Read the model definition and answer for the solid it produces. Units are mm, in the model's axes. A direction names the side the tool comes from. Coordinates: 2 decimals unless noted, no trailing zeros. Loops run counter-clockwise (first coordinate to the right, second up) from the corner with the lowest first, then second, coordinate; pieces in that order, holes last.
from build123d import *

# Parameters (mm, degrees)
SKETCH1_R           = 2.1209
SKETCH1_R_2         = 1.6002
BOSS_EXTRUDE1_DEPTH = 4.7625
CUT_EXTRUDE1_DEPTH  = 37.357096109
FILLET1_R           = 0.79375


with BuildPart() as part:
    # Sketch1 → Boss-Extrude1 (new body)
    with BuildSketch(Plane(origin=(0, 0, 0), x_dir=(0, 0, -1), z_dir=(1, 0, 0))):
        with BuildLine():
            ThreePointArc((-3.890248837, 27.252752244), (0, 34.7625), (3.890248837, 27.252752244))
            ThreePointArc((3.890248837, 27.252752244), (2.38125, 22.5), (3.890248837, 17.747247756))
            ThreePointArc((3.890248837, 17.747247756), (4.735348571, 15.507819022), (4.384317755, 13.140117187))
            ThreePointArc((4.384317755, 13.140117187), (4.159430641, 10.081636558), (5.845757006, 7.52015625))
            ThreePointArc((5.845757006, 7.52015625), (0, -9.525), (-5.845757006, 7.52015625))
            ThreePointArc((-5.845757006, 7.52015625), (-4.159430641, 10.081636558), (-4.384317755, 13.140117187))
            ThreePointArc((-4.384317755, 13.140117187), (-4.735348571, 15.507819022), (-3.890248837, 17.747247756))
            ThreePointArc((-3.890248837, 17.747247756), (-2.38125, 22.5), (-3.890248837, 27.252752244))
        make_face()
        with Locations(Location((0, 0, 0), (0, 0, 180))):
            Circle(SKETCH1_R, mode=Mode.SUBTRACT)
        with Locations(Location((0, 15, 0), (0, 0, 180))):
            Circle(SKETCH1_R_2, mode=Mode.SUBTRACT)
        with Locations(Location((0, 30, 0), (0, 0, 180))):
            Circle(SKETCH1_R_2, mode=Mode.SUBTRACT)
    extrude(amount=BOSS_EXTRUDE1_DEPTH)

    # Sketch2 → Cut-Extrude1 (cut, through all)
    with BuildSketch(Plane(origin=(4.7625, 0, 0), x_dir=(0, 0, -1), z_dir=(1, 0, 0))):
        with BuildLine():
            Line((-6.391057432, -4.707259409), (-4.102559861, -2.418761839))
            ThreePointArc((-4.102559861, -2.418761839), (-4.744354453, 0.41533971), (-3.619879359, 3.094814967))
            Line((-3.619879359, 3.094814967), (-5.263380295, 5.941442091))
            ThreePointArc((-5.263380295, 5.941442091), (-7.893363706, 0.835892131), (-6.391057432, -4.707259409))
        make_face()
        with BuildLine():
            Line((-2.418761839, -4.102559861), (-4.707259409, -6.391057432))
            ThreePointArc((-4.707259409, -6.391057432), (0, -7.9375), (4.707259409, -6.391057432))
            Line((4.707259409, -6.391057432), (2.418761839, -4.102559861))
            ThreePointArc((2.418761839, -4.102559861), (0, -4.7625), (-2.418761839, -4.102559861))
        make_face()
        with BuildLine():
            Line((-2.149945089, 6.898814128), (-0.870248702, 4.682314967))
            ThreePointArc((-0.870248702, 4.682314967), (0, 4.7625), (0.870248702, 4.682314967))
            Line((0.870248702, 4.682314967), (2.149945089, 6.898814128))
            ThreePointArc((2.149945089, 6.898814128), (1.320371493, 8.536647417), (0.889277805, 10.32126179))
            ThreePointArc((0.889277805, 10.32126179), (0, 10.2375), (-0.889277805, 10.32126179))
            ThreePointArc((-0.889277805, 10.32126179), (-1.320371493, 8.536647417), (-2.149945089, 6.898814128))
        make_face()
        with BuildLine():
            Line((6.391057432, -4.707259409), (4.102559861, -2.418761839))
            ThreePointArc((4.102559861, -2.418761839), (4.744354453, 0.41533971), (3.619879359, 3.094814967))
            Line((3.619879359, 3.094814967), (5.263380295, 5.941442091))
            ThreePointArc((5.263380295, 5.941442091), (7.893363706, 0.835892131), (6.391057432, -4.707259409))
        make_face()
    extrude(amount=-CUT_EXTRUDE1_DEPTH, mode=Mode.SUBTRACT)

    # Fillet1
    fillet1_edges = [part.edges().sort_by_distance(p)[0] for p in [
        (2.38125, -4.102559861, 2.418761839),
        (2.38125, -4.102559861, -2.418761839),
        (2.38125, -6.391057432, -4.707259409),
        (2.38125, -6.391057432, 4.707259409),
        (2.38125, 4.682314967, -0.870248702),
        (2.38125, 4.682314967, 0.870248702),
        (2.38125, 6.898814128, 2.149945089),
        (2.38125, 10.32126179, 0.889277805),
        (2.38125, 10.32126179, -0.889277805),
        (2.38125, 6.898814128, -2.149945089),
        (2.38125, 5.941442091, -5.263380295),
        (2.38125, -4.707259409, -6.391057432),
        (2.38125, -2.418761839, -4.102559861),
        (2.38125, 3.094814967, -3.619879359),
        (2.38125, -4.707259409, 6.391057432),
        (2.38125, 5.941442091, 5.263380295),
        (2.38125, 3.094814967, 3.619879359),
        (2.38125, -2.418761839, 4.102559861),
    ]]
    fillet(fillet1_edges, radius=FILLET1_R)


solid = part.part
Item 1: Which of the six approach directions +Z, -Z, +X, -X, +Y, -Y give full straight-line access (tool end or side, diameter ignored) to faces 3 (the face through (2.41, 4.29, 4.31)), 4 (the face through (2.35, 22.57, -2.38))?
Numbers:
face 3: +X, -X
face 4: -Z, +X, -X
Item 2: A cutting plane is placed at D-D on x = 2.1. Give the number of separate pieces and of enclosed holes in the cut face, then the cut area to 3 significant figures.
Numbers:
separate pieces: 1
enclosed holes: 7
area: 351 mm2
Item 3: Given pin 1 (1.5 mm diameter, centred on x = 1.5, y = -4.5, fed in from -Z), flat-ended and moving along its own axis, determine where the tip first touches the part or whether it passes through.
Numbers:
pin 1: stops at z = -8.76
Item 4: A cutting plane is placed at B-B on y = 0. Determine the outline of the cut face in (x, z) (1 decimal).
Numbers:
outline: (0, -9.5) - (4.8, -9.5) - (4.8, -7.9) - (0, -7.9) - close; (0, -4.8) - (4.8, -4.8) - (4.8, -2.1) - (0, -2.1) - close; (0, 2.1) - (4.8, 2.1) - (4.8, 4.8) - (0, 4.8) - close; (0, 7.9) - (4.8, 7.9) - (4.8, 9.5) - (0, 9.5) - close
Item 5: Find the intervals of material crossed by line 1 along Z through (x, y) = (1.4, 15); line 2 along Z through (x, y) = (2.25, 1.5); line 3 along Y through (x, z) = (1.35, -3), in increasing order.
Numbers:
line 1: z = -4.76 to -1.6, 1.6 to 4.76
line 2: z = -9.41 to -7.79, -4.52 to -1.5, 1.5 to 4.52, 7.79 to 9.41
line 3: y = -9.04 to -7.35, -4.68 to 19.37, 25.63 to 33.7
Item 6: A cutting plane is placed at C-C on z = 3.25. Determine the outline of the cut face in (x, y).
Numbers:
outline: (0, -8.95) - (4.76, -8.95) - (4.76, -7.24) - (0, -7.24) - close; (0, -4.93) - (4.76, -4.93) - (4.76, 18.82) - (0, 18.82) - close; (0, 26.18) - (4.76, 26.18) - (4.76, 33.48) - (0, 33.48) - close
Item 7: Determine the mould class of faces 1 (the face through (2.35, -9.52, -0.33)), 2 (the face through (2.35, -4.29, -2.4)) for opening direction Y: released by +Y, released by -Y, zero draft, split by the parting line, or undercut.
Numbers:
face 1: split by the parting line
face 2: undercut
Item 8: A cutting plane is placed at A-A on y = 30. Determine the outline of the cut face in (x, z), then the cut area to 3 significant figures.
Numbers:
outline: (0, -4.76) - (4.76, -4.76) - (4.76, -1.6) - (0, -1.6) - close; (0, 1.6) - (4.76, 1.6) - (4.76, 4.76) - (0, 4.76) - close
area: 30.1 mm2
